from build123d import *

# Parameters (mm, degrees)
BOSS_EXTRUDE1_DEPTH     = 504
CUT_EXTRUDE4_REACH      = 514.328
CUT_EXTRUDE4_END_RADIUS = 90
SKETCH6_R               = 2.5
CUT_EXTRUDE2_REACH      = 516.263
CUT_EXTRUDE2_END_RADIUS = 90
SKETCH3_R               = 2.5
CUT_EXTRUDE3_REACH      = 516.263
CUT_EXTRUDE3_END_RADIUS = 90
SKETCH5_R               = 2.5
LPATTERN2_COUNT         = 2
LPATTERN2_PITCH         = 491
CUT_EXTRUDE5_DEPTH      = 13
CUT_EXTRUDE6_START      = -13
CUT_EXTRUDE6_DEPTH      = 13
BODY_MOVE_COPY1_ANGLE   = 180


with BuildPart() as part:
    # Sketch1 → Boss-Extrude1 (new body)
    with BuildSketch(Plane(origin=(0, 0, 0), x_dir=(1, 0, 0), z_dir=(0, 1, 0))):
        with BuildLine():
            Line((0, 92), (0, 90))
            ThreePointArc((0, 90), (63.639610307, 63.639610307), (90, 0))
            Line((90, 0), (92, 0))
            ThreePointArc((92, 0), (65.053823869, 65.053823869), (0, 92))
        make_face()
    extrude(amount=BOSS_EXTRUDE1_DEPTH)

    # Cut-Extrude4: up to this cylinder (the profile starts outside it)
    cut_extrude4_end = Plane(origin=(0, 6.5, 0), z_dir=(0, -1, 0)) * Cylinder(CUT_EXTRUDE4_END_RADIUS, 1209.656, mode=Mode.PRIVATE)
    # Sketch6 → Cut-Extrude4 (cut, up to the surface)
    with BuildSketch(Plane(origin=(65.053823869, 0, -65.053823869), x_dir=(-0.7071067811865486, 0, -0.7071067811865465), z_dir=(0.7071067811865465, 0, -0.7071067811865486)), mode=Mode.PRIVATE) as cut_extrude4_sk1:
        with Locations((0, 6.5)):
            Circle(SKETCH6_R)
    cut_extrude4_tool1 = extrude(cut_extrude4_sk1.sketch, amount=-CUT_EXTRUDE4_REACH, mode=Mode.PRIVATE) - cut_extrude4_end
    cut_extrude4 = cut_extrude4_tool1.solids().sort_by_distance((65.053824, 6.5, -65.053824))[0]
    add(cut_extrude4, mode=Mode.SUBTRACT)

    # Cut-Extrude2: up to this cylinder (the profile starts outside it)
    cut_extrude2_end = Plane(origin=(0, 6.5, 0), z_dir=(0, -1, 0)) * Cylinder(CUT_EXTRUDE2_END_RADIUS, 1213.526, mode=Mode.PRIVATE)
    # Sketch3 → Cut-Extrude2 (cut, up to the surface)
    with BuildSketch(Plane(origin=(84.996916991, 0, -35.206875778), x_dir=(-0.38268343236509045, 0, -0.9238795325112865), z_dir=(0.9238795325112865, 0, -0.38268343236509045)), mode=Mode.PRIVATE) as cut_extrude2_sk1:
        with Locations((0, 6.5)):
            Circle(SKETCH3_R)
    cut_extrude2_tool1 = extrude(cut_extrude2_sk1.sketch, amount=-CUT_EXTRUDE2_REACH, mode=Mode.PRIVATE) - cut_extrude2_end
    cut_extrude2 = cut_extrude2_tool1.solids().sort_by_distance((84.996917, 6.5, -35.206876))[0]
    add(cut_extrude2, mode=Mode.SUBTRACT)

    # Cut-Extrude3: up to this cylinder (the profile starts outside it)
    cut_extrude3_end = Plane(origin=(0, 6.5, 0), z_dir=(0, -1, 0)) * Cylinder(CUT_EXTRUDE3_END_RADIUS, 1213.526, mode=Mode.PRIVATE)
    # Sketch5 → Cut-Extrude3 (cut, up to the surface)
    with BuildSketch(Plane(origin=(35.206875778, 0, -84.996916991), x_dir=(-0.9238795325112878, 0, -0.3826834323650876), z_dir=(0.3826834323650876, 0, -0.9238795325112878)), mode=Mode.PRIVATE) as cut_extrude3_sk1:
        with Locations((0, 6.5)):
            Circle(SKETCH5_R)
    cut_extrude3_tool1 = extrude(cut_extrude3_sk1.sketch, amount=-CUT_EXTRUDE3_REACH, mode=Mode.PRIVATE) - cut_extrude3_end
    cut_extrude3 = cut_extrude3_tool1.solids().sort_by_distance((35.206876, 6.5, -84.996917))[0]
    add(cut_extrude3, mode=Mode.SUBTRACT)

    # LPattern2: Cut-Extrude4, Cut-Extrude2, Cut-Extrude3 ×2
    with Locations(*[(0, i * LPATTERN2_PITCH, 0) for i in range(1, LPATTERN2_COUNT)]):
        add(cut_extrude4, mode=Mode.SUBTRACT)
        add(cut_extrude2, mode=Mode.SUBTRACT)
        add(cut_extrude3, mode=Mode.SUBTRACT)

    # Sketch7 → Cut-Extrude5 (cut)
    with BuildSketch(Plane.XZ):
        with BuildLine():
            Line((76.447375943, -51.183969281), (74.784435976, -50.072828318))
            ThreePointArc((74.784435976, -50.072828318), (63.639610307, -63.639610307), (50.072828318, -74.784435976))
            Line((50.072828318, -74.784435976), (51.183969281, -76.447375943))
            ThreePointArc((51.183969281, -76.447375943), (65.053823869, -65.053823869), (76.447375943, -51.183969281))
        make_face()
    extrude(amount=-CUT_EXTRUDE5_DEPTH, mode=Mode.SUBTRACT)

    # Sketch9 → Cut-Extrude6 (cut)
    with BuildSketch(Plane(origin=(0, 504, 0), x_dir=(1, 0, 0), z_dir=(0, 1, 0)).offset(CUT_EXTRUDE6_START)):
        with BuildLine():
            ThreePointArc((0, 90), (26.125620953, 86.124630216), (50.001320972, 74.832265107))
            Line((50.001320972, 74.832265107), (51.112461438, 76.495204332))
            ThreePointArc((51.112461438, 76.495204332), (26.706190307, 88.038510887), (0, 92))
            Line((0, 92), (0, 90))
        make_face()
        with BuildLine():
            ThreePointArc((74.832265107, 50.001320972), (86.124630216, 26.125620953), (90, 0))
            Line((90, 0), (92, 0))
            ThreePointArc((92, 0), (88.038510887, 26.706190307), (76.495204332, 51.112461438))
            Line((76.495204332, 51.112461438), (74.832265107, 50.001320972))
        make_face()
    extrude(amount=CUT_EXTRUDE6_DEPTH, mode=Mode.SUBTRACT)


with BuildPart() as part_1:
    # Body-Move/Copy1: moved
    add(part.part.moved(Location((0, 0, 0))).rotate(Axis((0, 252, 0), (0.7071067811865488, -4.937700262164522e-15, -0.7071067811865462)), BODY_MOVE_COPY1_ANGLE))


solid = part_1.part
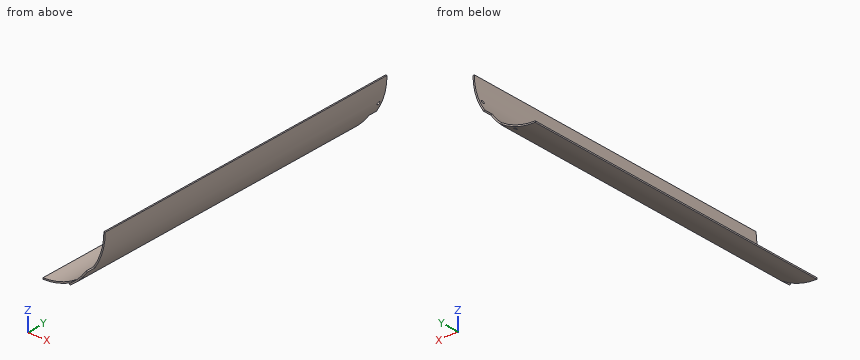
Geometry check sheet. Reference: the model listing, model coordinates, mm. Give positions to 0.01 mm unless a question says otherwise; leave off trailing zeros. Write each loop counter-clockwise with the first axis right and the second up, starting at its lowest first coordinate (ties: lowest second). Pieces come first, ordered by that corner, then holes.
1) Cross-section at A-A (y = 188.5). Record the boundary of the cut face in (x, z), plus the area to 3 significant figures.
Values follow:
outline: (0, -92) arc R92 ccw to (92, 0) - (90, 0) arc R90 cw to (0, -90) - close
area: 286 mm2
2) Thickness scan on line 1 (X direction, y = 25, z = -59); line 2 (Z direction, x = 23, y = 262); line 3 (X direction, y = 402, z = -42). Record the ranges inside material, lowest first.
Values follow:
line 1: x = 67.96 to 70.59
line 2: z = -89.08 to -87.01
line 3: x = 79.6 to 81.85
3) Go/stop test with flat-tipped pins: pin 1 Ø12 at (x, y) = (20, 349) entering from +Z; pin 2 Ø10 at (x, y) = (15.5, 298) entering from -Z; pin 3 Ø1 at (y, z) = (392.5, -81.5) entering from -X. Record where each tip stops, or that it passes through.
Values follow:
pin 1: stops at z = -86.16
pin 2: stops at z = -91.4
pin 3: stops at x = 37.09
4) Cross-section at B-B (x = 14.5). Record the boundary of the cut face in (y, z).
Values follow:
outline: (13, -90.85) - (504, -90.85) - (504, -88.82) - (13, -88.82) - close
